```python
from build123d import *

# Parameters (mm, degrees)
BOSS_EXTRUDE1_DEPTH = 15
SKETCH2_R           = 1.75
CUT_EXTRUDE1_DEPTH  = 6


with BuildPart() as part:
    # Sketch1 → Boss-Extrude1 (new body)
    with BuildSketch(Plane(origin=(0, 0, 0), x_dir=(1, 0, 0), z_dir=(0, 1, 0))):
        with BuildLine():
            Line((-35.7, -7.2), (-35.7, -12.2))
            Line((-35.7, -12.2), (-12.7, -12.2))
            Line((-12.7, -12.2), (-12.7, 0))
            ThreePointArc((-12.7, 0), (0, 12.7), (12.7, 0))
            Line((12.7, 0), (12.7, -12.2))
            Line((12.7, -12.2), (35.7, -12.2))
            Line((35.7, -12.2), (35.7, -7.2))
            Line((35.7, -7.2), (17.7, -7.2))
            Line((17.7, -7.2), (17.7, 0))
            ThreePointArc((17.7, 0), (0, 17.7), (-17.7, 0))
            Line((-17.7, 0), (-17.7, -7.2))
            Line((-17.7, -7.2), (-35.7, -7.2))
        make_face()
    extrude(amount=BOSS_EXTRUDE1_DEPTH)

    # Sketch2 → Cut-Extrude1 (cut, through all)
    with BuildSketch(Plane(origin=(0, 0, 7.2), x_dir=(-1, 0, 0), z_dir=(0, 0, -1))):
        with Locations((-30, 7.5)):
            Circle(SKETCH2_R)
        with Locations((30, 7.5)):
            Circle(SKETCH2_R)
    extrude(amount=-CUT_EXTRUDE1_DEPTH, mode=Mode.SUBTRACT)


solid = part.part
```
Source: CAD feature listing. Evaluate the final solid. Frame: model axes, mm. A direction names the side the tool comes from. Give positions to 0.01 mm unless a question says otherwise; leave off trailing zeros. Loops run counter-clockwise (first coordinate to the right, second up) from the corner with the lowest first, then second, coordinate; pieces in that order, holes last. Notation, with made-up numbers: (-1, -2) - (52, -2) arc R23 ccw to (52, 12) - close; hole circle Ø11 at (89.5, 43). An arc over 180 degrees is marked (long way). Use CSV: the item, a comma, the result in double quotes. Start each with the question number.
1. Section A-A (z = 2.75). Output: boundary loops of the cut face in (x, y).
2. Section B-B (y = 7.5). Output: boundary loops of the cut face in (x, z).
3. Section C-C (x = -30). Output: boundary loops of the cut face in (y, z), then the cut area to 3 significant figures.
4. Draft query along X for faces 5 (the flat face through (17.7, 7, 4)), 6 (the cylindrical face through (-0.279, 7.395, -12.697)), 7 (the flat face through (24, 7, 12.2)). Return one class per face: +X half, -X half, draft (parallel to the pull), parting line (faces both ways), or undercut.
5. Ray query, L1, parallel to Y at x = 30, z = 10.05; L2, parallel to X at y = 5.5, z = 2.5; L3, parallel to X at y = 5.25, z = 10. Return the intervals inside material, ascending.
6. Reachability of faces 1 (the flat face through (27, 7, 7.2)), 2 (the flat face through (-17.7, 7, 4)), 3 (the flat face through (12.7, 7, 6)), 4 (the flat face through (35.7, 7, 10)) from +Z, -Z, +X, -X, +Y, -Y: full face, straight path, thin tool, end or side. Return the list, or none.
7. Section D-D (y = 1.25). Output: boundary loops of the cut face in (x, z).
8. Pin query (flat end, axial travel): pin 1 (4 mm diameter, centred on x = 17, y = 3, fed in from -Z); pin 2 (6 mm diameter, centred on y = 7.5, z = 4, fed in from -X); pin 3 (5 mm diameter, centred on x = -17, y = 13.5, fed in from -Z); pin 4 (5.5 mm diameter, centred on x = 30, y = 7.5, fed in from +Z). Return the tip coordinate at first contact, or that it passes through.
Response:
1,outline,"(-17.7, 0) - (-12.7, 0) - (-12.7, 15) - (-17.7, 15) - close; (12.7, 0) - (17.7, 0) - (17.7, 15) - (12.7, 15) - close"
2,outline,"(-35.7, 7.2) - (-31.75, 7.2) - (-31.75, 12.2) - (-35.7, 12.2) - close; (-28.25, 7.2) - (-17.7, 7.2) - (-17.7, 0) arc R17.7 ccw to (17.7, 0) - (17.7, 7.2) - (28.25, 7.2) - (28.25, 12.2) - (12.7, 12.2) - (12.7, 0) arc R12.7 cw to (-12.7, 0) - (-12.7, 12.2) - (-28.25, 12.2) - close; (31.75, 7.2) - (35.7, 7.2) - (35.7, 12.2) - (31.75, 12.2) - close"
3,outline,"(0, 7.2) - (5.75, 7.2) - (5.75, 12.2) - (0, 12.2) - close; (9.25, 7.2) - (15, 7.2) - (15, 12.2) - (9.25, 12.2) - close"
3,area,"57.5 mm²"
4,face 5,"+X half"
4,face 6,"undercut"
4,face 7,"draft"
5,L1,"0 to 5.75, 9.25 to 15"
5,L2,"-17.7 to -12.7, 12.7 to 17.7"
5,L3,"-35.7 to -12.7, 12.7 to 35.7"
6,face 1,"-Z, +X, +Y, -Y"
6,face 2,"-Z, -X, +Y, -Y"
6,face 3,"+Z, +Y, -Y"
6,face 4,"+Z, -Z, +X, +Y, -Y"
7,outline,"(-35.7, 7.2) - (-17.7, 7.2) - (-17.7, 0) arc R17.7 ccw to (17.7, 0) - (17.7, 7.2) - (35.7, 7.2) - (35.7, 12.2) - (12.7, 12.2) - (12.7, 0) arc R12.7 cw to (-12.7, 0) - (-12.7, 12.2) - (-35.7, 12.2) - close"
8,pin 1,"z = -9.4"
8,pin 2,"x = -17.7"
8,pin 3,"z = -10.15"
8,pin 4,"z = 12.2"
